```python
from build123d import *

# Parameters (mm, degrees)
SKETCH1_W           = 65.359412811
SKETCH1_H           = 25.4
BOSS_EXTRUDE1_DEPTH = 36.322
SKETCH4_W           = 50.419
SKETCH4_H           = 33.02
SKETCH4_W_2         = 2.9972
SKETCH4_H_2         = 22.86
CUT_EXTRUDE1_DEPTH  = 78.438347632
CUT_EXTRUDE2_REACH  = 80.97
SKETCH5_R           = 2.76225
CUT_EXTRUDE3_REACH  = 80.97
SKETCH6_R           = 0.9525
CUT_EXTRUDE5_REACH  = 80.97
SKETCH7_R           = 6.604
SKETCH7_R_2         = 0.9525
CUT_EXTRUDE6_REACH  = 73.327
FILLET1_R           = 12.7
FILLET2_R           = 2.54
SKETCH10_W          = 19.05
SKETCH10_H          = 11.43
CUT_EXTRUDE7_DEPTH  = 78.438347679


with BuildPart() as part:
    # Sketch1 → Boss-Extrude1 (new body)
    with BuildSketch(Plane.XY):
        with Locations((-30.820293595, 12.7)):
            Rectangle(SKETCH1_W, SKETCH1_H)
    extrude(amount=BOSS_EXTRUDE1_DEPTH)

    # Sketch4 → Cut-Extrude1 (cut, through all)
    with BuildSketch(Plane(origin=(0, 25.4, 0), x_dir=(1, 0, 0), z_dir=(0, 1, 0))):
        with Locations((-32.824287189, -19.812)):
            Rectangle(SKETCH4_W, SKETCH4_H)
        with Locations((-4.211187189, -24.892)):
            Rectangle(SKETCH4_W_2, SKETCH4_H_2)
    extrude(amount=-CUT_EXTRUDE1_DEPTH, mode=Mode.SUBTRACT)

    # Sketch5 → Cut-Extrude2 (cut, up to next)
    with BuildSketch(Plane(origin=(1.859412811, 0, 0), x_dir=(0, 0, -1), z_dir=(1, 0, 0)), mode=Mode.PRIVATE) as cut_extrude2_sk1:
        with Locations(Location((-24.892, 12.7, 0), (0, 0, 90))):
            Circle(SKETCH5_R)
    cut_extrude2_tool1 = extrude(cut_extrude2_sk1.sketch, amount=-CUT_EXTRUDE2_REACH, mode=Mode.PRIVATE) & part.part
    add(cut_extrude2_tool1.solids().sort_by_distance((1.859413, 12.7, 24.892))[0], mode=Mode.SUBTRACT)

    # Cut-Extrude3: up to this face of the body (flat: up to its plane)
    cut_extrude3_end = Plane(part.part.faces().sort_by_distance((-7.614787189, 12.7, 19.812))[0])
    # Sketch6 → Cut-Extrude3 (cut, up to the picked face)
    with BuildSketch(Plane(origin=(1.859412811, 0, 0), x_dir=(0, 0, -1), z_dir=(1, 0, 0)), mode=Mode.PRIVATE) as cut_extrude3_sk1:
        with Locations(Location((-24.892, 12.7, 0), (0, 0, 90))):
            Circle(SKETCH6_R)
    cut_extrude3_tool1 = split(extrude(cut_extrude3_sk1.sketch, amount=-CUT_EXTRUDE3_REACH, mode=Mode.PRIVATE), bisect_by=cut_extrude3_end, keep=Keep.BOTH, mode=Mode.PRIVATE)
    # Sketch6 → Cut-Extrude3 (cut, up to the picked face)
    with BuildSketch(Plane(origin=(1.859412811, 0, 0), x_dir=(0, 0, -1), z_dir=(1, 0, 0)), mode=Mode.PRIVATE) as cut_extrude3_sk2:
        with Locations(Location((-24.892, 19.7, 0), (0, 0, 90))):
            Circle(SKETCH6_R)
    cut_extrude3_tool2 = split(extrude(cut_extrude3_sk2.sketch, amount=-CUT_EXTRUDE3_REACH, mode=Mode.PRIVATE), bisect_by=cut_extrude3_end, keep=Keep.BOTH, mode=Mode.PRIVATE)
    # Sketch6 → Cut-Extrude3 (cut, up to the picked face)
    with BuildSketch(Plane(origin=(1.859412811, 0, 0), x_dir=(0, 0, -1), z_dir=(1, 0, 0)), mode=Mode.PRIVATE) as cut_extrude3_sk3:
        with Locations(Location((-17.892, 12.7, 0), (0, 0, 90))):
            Circle(SKETCH6_R)
    cut_extrude3_tool3 = split(extrude(cut_extrude3_sk3.sketch, amount=-CUT_EXTRUDE3_REACH, mode=Mode.PRIVATE), bisect_by=cut_extrude3_end, keep=Keep.BOTH, mode=Mode.PRIVATE)
    # Sketch6 → Cut-Extrude3 (cut, up to the picked face)
    with BuildSketch(Plane(origin=(1.859412811, 0, 0), x_dir=(0, 0, -1), z_dir=(1, 0, 0)), mode=Mode.PRIVATE) as cut_extrude3_sk4:
        with Locations(Location((-24.892, 5.7, 0), (0, 0, 90))):
            Circle(SKETCH6_R)
    cut_extrude3_tool4 = split(extrude(cut_extrude3_sk4.sketch, amount=-CUT_EXTRUDE3_REACH, mode=Mode.PRIVATE), bisect_by=cut_extrude3_end, keep=Keep.BOTH, mode=Mode.PRIVATE)
    # Sketch6 → Cut-Extrude3 (cut, up to the picked face)
    with BuildSketch(Plane(origin=(1.859412811, 0, 0), x_dir=(0, 0, -1), z_dir=(1, 0, 0)), mode=Mode.PRIVATE) as cut_extrude3_sk5:
        with Locations(Location((-31.892, 12.7, 0), (0, 0, 90))):
            Circle(SKETCH6_R)
    cut_extrude3_tool5 = split(extrude(cut_extrude3_sk5.sketch, amount=-CUT_EXTRUDE3_REACH, mode=Mode.PRIVATE), bisect_by=cut_extrude3_end, keep=Keep.BOTH, mode=Mode.PRIVATE)
    add(cut_extrude3_tool1.solids().sort_by(Axis((1.859413, 12.7, 24.892), (-1, 0, 0)))[0], mode=Mode.SUBTRACT)
    add(cut_extrude3_tool2.solids().sort_by(Axis((1.859413, 19.7, 24.892), (-1, 0, 0)))[0], mode=Mode.SUBTRACT)
    add(cut_extrude3_tool3.solids().sort_by(Axis((1.859413, 12.7, 17.892), (-1, 0, 0)))[0], mode=Mode.SUBTRACT)
    add(cut_extrude3_tool4.solids().sort_by(Axis((1.859413, 5.7, 24.892), (-1, 0, 0)))[0], mode=Mode.SUBTRACT)
    add(cut_extrude3_tool5.solids().sort_by(Axis((1.859413, 12.7, 31.892), (-1, 0, 0)))[0], mode=Mode.SUBTRACT)

    # Sketch7 → Cut-Extrude5 (cut, up to next)
    with BuildSketch(Plane.ZY.offset(63.5), mode=Mode.PRIVATE) as cut_extrude5_sk1:
        with Locations((24.892, 12.7)):
            Circle(SKETCH7_R)
        with Locations(Location((24.892, 12.7, 0), (0, 0, 90))):
            Circle(SKETCH7_R_2, mode=Mode.SUBTRACT)
    cut_extrude5_tool1 = extrude(cut_extrude5_sk1.sketch, amount=-CUT_EXTRUDE5_REACH, mode=Mode.PRIVATE) & part.part
    # Sketch7 → Cut-Extrude5 (cut, up to next)
    with BuildSketch(Plane.ZY.offset(63.5), mode=Mode.PRIVATE) as cut_extrude5_sk2:
        with Locations(Location((24.892, 12.7, 0), (0, 0, 90))):
            Circle(SKETCH7_R_2)
    cut_extrude5_tool2 = extrude(cut_extrude5_sk2.sketch, amount=-CUT_EXTRUDE5_REACH, mode=Mode.PRIVATE) & part.part
    add(cut_extrude5_tool1.solids().sort_by_distance((-63.5, 12.7, 18.474789))[0], mode=Mode.SUBTRACT)
    add(cut_extrude5_tool2.solids().sort_by_distance((-63.5, 12.7, 24.892))[0], mode=Mode.SUBTRACT)

    # Sketch8 → Cut-Extrude6 (cut, up to next)
    with BuildSketch(Plane.ZY.offset(7.614787189), mode=Mode.PRIVATE) as cut_extrude6_sk1:
        with BuildLine():
            Line((36.322, 17.2), (23.622, 17.2))
            ThreePointArc((23.622, 17.2), (19.122, 12.7), (23.622, 8.2))
            Line((23.622, 8.2), (36.322, 8.2))
            Line((36.322, 8.2), (36.322, 17.2))
        make_face()
    cut_extrude6_tool1 = extrude(cut_extrude6_sk1.sketch, amount=-CUT_EXTRUDE6_REACH, mode=Mode.PRIVATE) & part.part
    add(cut_extrude6_tool1.solids().sort_by_distance((-7.614787, 12.7, 28.173785))[0], mode=Mode.SUBTRACT)

    # Fillet1
    # the kernel refuses this fillet: 12.7 mm, written as the material it takes off along each edge
    with BuildSketch(Plane(origin=(-63.5, 0, 36.322), x_dir=(0, 0, -1), z_dir=(1, 0, 0))) as fillet1_piece_1:
        with BuildLine():
            CenterArc((FILLET1_R, FILLET1_R), FILLET1_R, 180, 90)
            Line((0, FILLET1_R), (-FILLET1_R * 0.02, FILLET1_R))
            Line((-FILLET1_R * 0.02, FILLET1_R), (-FILLET1_R * 0.02, -FILLET1_R * 0.02))
            Line((-FILLET1_R * 0.02, -FILLET1_R * 0.02), (FILLET1_R, -FILLET1_R * 0.02))
            Line((FILLET1_R, -FILLET1_R * 0.02), (FILLET1_R, 0))
        make_face()
    extrude(amount=5.466212811, mode=Mode.SUBTRACT)
    with BuildSketch(Plane(origin=(-7.614787189, 0, 36.322), x_dir=(0, 0, -1), z_dir=(1, 0, 0)), Plane(origin=(-5.709787189, 25.4, 36.322), x_dir=(0, 0, -1), z_dir=(-1, 0, 0))) as fillet1_piece_2:
        with BuildLine():
            CenterArc((11.876026271, 12.7), FILLET1_R, 200.752430643, 69.247569357)
            Line((0, 8.2), (-0.237520525, 8.11))
            ThreePointArc((-0.237520525, 8.11), (-0.254, 4.1), (-0.254, 0))
            Line((-0.254, 0), (0, -0.254))
            Line((0, -0.254), (11.876026271, -0.254))
            Line((11.876026271, -0.254), (11.876026271, 0))
        make_face()
    extrude(amount=1.905, mode=Mode.SUBTRACT)
    with BuildSketch(Plane(origin=(-2.712587189, 0, 36.322), x_dir=(0, 0, -1), z_dir=(1, 0, 0))) as fillet1_piece_3:
        with BuildLine():
            CenterArc((FILLET1_R, FILLET1_R), FILLET1_R, 180, 90)
            Line((0, FILLET1_R), (-FILLET1_R * 0.02, FILLET1_R))
            Line((-FILLET1_R * 0.02, FILLET1_R), (-FILLET1_R * 0.02, -FILLET1_R * 0.02))
            Line((-FILLET1_R * 0.02, -FILLET1_R * 0.02), (FILLET1_R, -FILLET1_R * 0.02))
            Line((FILLET1_R, -FILLET1_R * 0.02), (FILLET1_R, 0))
        make_face()
    extrude(amount=4.572, mode=Mode.SUBTRACT)
    with BuildSketch(Plane(origin=(1.859412811, 25.4, 36.322), x_dir=(0, -1, 0), z_dir=(-1, 0, 0))) as fillet1_piece_4:
        with BuildLine():
            CenterArc((FILLET1_R, -FILLET1_R), FILLET1_R, 90, 90)
            Line((0, -FILLET1_R), (-FILLET1_R * 0.02, -FILLET1_R))
            Line((-FILLET1_R * 0.02, -FILLET1_R), (-FILLET1_R * 0.02, FILLET1_R * 0.02))
            Line((-FILLET1_R * 0.02, FILLET1_R * 0.02), (FILLET1_R, FILLET1_R * 0.02))
            Line((FILLET1_R, FILLET1_R * 0.02), (FILLET1_R, 0))
        make_face()
    extrude(amount=4.572, mode=Mode.SUBTRACT)
    with BuildSketch(Plane(origin=(-58.033787189, 25.4, 36.322), x_dir=(0, -1, 0), z_dir=(-1, 0, 0))) as fillet1_piece_5:
        with BuildLine():
            CenterArc((FILLET1_R, -FILLET1_R), FILLET1_R, 90, 90)
            Line((0, -FILLET1_R), (-FILLET1_R * 0.02, -FILLET1_R))
            Line((-FILLET1_R * 0.02, -FILLET1_R), (-FILLET1_R * 0.02, FILLET1_R * 0.02))
            Line((-FILLET1_R * 0.02, FILLET1_R * 0.02), (FILLET1_R, FILLET1_R * 0.02))
            Line((FILLET1_R, FILLET1_R * 0.02), (FILLET1_R, 0))
        make_face()
    extrude(amount=5.466212811, mode=Mode.SUBTRACT)

    # Fillet2
    fillet2_edges = [part.edges().sort_by_distance(p)[0] for p in [
        (-6.662287189, 8.2, 36.322),
        (-6.662287189, 17.2, 36.322),
        (-63.5, 0, 11.811),
        (1.859412811, 0, 11.811),
        (-63.5, 25.4, 11.811),
        (-63.5, 21.680256121, 32.602256121),
        (-63.5, 3.719743879, 32.602256121),
        (1.859412811, 25.4, 11.811),
        (1.859412811, 21.680256121, 32.602256121),
        (1.859412811, 3.719743879, 32.602256121),
    ]]
    fillet(fillet2_edges, radius=FILLET2_R)

    # Sketch10 → Cut-Extrude7 (cut, through all)
    with BuildSketch(Plane(origin=(0, 0, 0), x_dir=(-1, 0, 0), z_dir=(0, 0, -1))):
        with Locations((32.007264904, 8.255)):
            Rectangle(SKETCH10_W, SKETCH10_H)
    extrude(amount=-CUT_EXTRUDE7_DEPTH, mode=Mode.SUBTRACT)


solid = part.part
```
Work out the finished part from the listing and answer in its coordinate system (mm). A direction names the side the tool comes from. Give positions to 0.01 mm unless a question says otherwise; leave off trailing zeros. Order: outer loops, then holes, each group sorted by start corner. A loop starts at its lowest first (then second) coordinate and runs counter-clockwise, first axis right, second up.
1. Straight lines are drawn through the part: L1, parallel to X at y = 3.5, z = 18; L2, parallel to Z at x = -6.3, y = 19.7; L3, parallel to X at y = 15.25, z = 6.5. For each, find the intervals that lie inside material, in ascending order.
Result sheet:
L1: x = -63.5 to -58.03, -7.61 to -5.71, -2.71 to 1.86
L2: z = 0 to 23.94, 25.84 to 34.31
L3: x = -63.5 to -58.03, -7.61 to 1.86
2. Section C-C, the plane z = 28.5 is taken. Give the number of separate pieces and of enclosed holes in the cut face, and give its area (3 significant figures).
Result sheet:
separate pieces: 5
enclosed holes: 0
area: 198 mm2
3. Section A-A, the plane z = 15.5 is taken. Determine the outline of the cut face in (x, y), and give its area (3 significant figures).
Result sheet:
outline: (-63.5, 2.54) arc R2.54 ccw to (-60.96, 0) - (-58.03, 0) - (-58.03, 25.4) - (-60.96, 25.4) arc R2.54 ccw to (-63.5, 22.86) - close; (-7.61, 0) - (-5.71, 0) - (-5.71, 25.4) - (-7.61, 25.4) - close; (-2.71, 0) - (-0.68, 0) arc R2.54 ccw to (1.86, 2.54) - (1.86, 22.86) arc R2.54 ccw to (-0.68, 25.4) - (-2.71, 25.4) - close
area: 298 mm2
4. Each of these flat-tipped pins is pushed along its axis until it touches: P1, Ø8, axis at x = -37.5, y = 16.5, coming from the +Z side; P2, Ø2, axis at x = -6.5, z = 27, coming from the +Y side; P3, Ø1.7, axis at y = 19.7, z = 24.892, coming from the +X side. Where does it stop, or does it pass through?
Result sheet:
P1: stops at z = 3.3
P2: stops at y = 25.3
P3: stops at x = -58.03
5. Section B-B, the plane x = -39 is taken. Determine the outline of the cut face in (y, z), and give its area (3 significant figures).
Result sheet:
outline: (0, 0) - (2.54, 0) - (2.54, 3.3) - (0, 3.3) - close; (13.97, 0) - (25.4, 0) - (25.4, 3.3) - (13.97, 3.3) - close
area: 46.1 mm2
6. The mould has two halves that part along Z. Classify faces 1 (the cylindrical face through (-0.39, 19, 25.54)), 2 (the flat face through (-22.482, 8, 2)), 3 (the cylindrical face through (-6.676, 1.044, 29.488)): released by +Z, released by -Z, zero draft, split by the parting line, or undercut.
Result sheet:
face 1: undercut
face 2: zero draft
face 3: released by +Z
7. For faces 4 (the cylindrical face through (-0.39, 11.75, 17.93)), 5 (the cylindrical face through (-6.649, 24.356, 29.488)), 6 (the flat face through (-7, 8.2, 28)), 7 (the flat face through (-58.034, 13, 16)), determine the directions among +Z, -Z, +X, -X, +Y, -Y from which every point of the face is accessible in a straight line to the end or side of a thin tool.
Result sheet:
face 4: +X
face 5: +Z, +X, -X, +Y
face 6: +Z
face 7: +Z, +Y, -Y
